```python
from build123d import *

# Parameters (mm, degrees)
F0_W      = 298.5
F0_H      = 130
F1_DEPTH  = 14
F2_W      = 20
F2_H      = 10
F3_DEPTH  = 130
F4_W      = 11
F4_H      = 16
F5_DEPTH  = 130
F6_W      = 39.1095238095
F6_H      = 26.9544340008
F6_W_2    = 43.7704761905
F6_H_2    = 58.0455659992
F7_DEPTH  = 25
F8_R      = 2.5
F9_DEPTH  = 25
F10_R     = 2.5
F11_DEPTH = 318.501
F12_SIZE  = 3.49999
F14_W     = 276.5
F14_H     = 15
F13_DEPTH = 25


# Not quite as in the source:
# - a fillet or chamfer is up to 0.001 mm smaller than in the source, because OpenCascade refuses the exact size
# - a feature names something its author has since deleted; it is built from what else it names


with BuildPart() as f1:
    # F0 (on Front) → F1 (new body)
    with BuildSketch(Plane.XZ):
        with Locations((149.25, 65)):
            Rectangle(F0_W, F0_H)
    extrude(amount=F1_DEPTH)

    # F2 (on face) → F3 (join, through all)
    with BuildSketch(Plane.XY.offset(130)):
        with Locations((308.5, -9)):
            Rectangle(F2_W, F2_H)
        with Locations((-10, -9)):
            Rectangle(F2_W, F2_H)
    extrude(amount=-F3_DEPTH)

    # F4 (on face) → F5 (join, through all)
    with BuildSketch(Plane.XY.offset(130)):
        with Locations((5.5, 8)):
            Rectangle(F4_W, F4_H)
        with Locations((293, 8)):
            Rectangle(F4_W, F4_H)
    extrude(amount=-F5_DEPTH)

    # F6 (on face) → F7 (cut)
    with BuildSketch(Plane.XZ.offset(14)):
        Polygon((51.37, 120), (51.37, 93.0455659992), (36.37, 93.0455659992), (36.3699999999, 56.9544340008), (90.4795238095, 56.9544340008), (90.4795238095, 120), align=None)
        with Locations((70.9247619048, 28.4772170004)):
            Rectangle(F6_W, F6_H)
        with Locations((127.3647619048, 44.0227829996)):
            Rectangle(F6_W_2, F6_H_2)
        with Locations((171.1352380952, 44.0227829996)):
            Rectangle(F6_W_2, F6_H_2)
        with Locations((127.3647619048, 106.5227829996)):
            Rectangle(F6_W_2, F6_H)
        with Locations((171.1352380952, 106.5227829996)):
            Rectangle(F6_W_2, F6_H)
        Polygon((247.1300000001, 120), (208.0204761905, 120), (208.0204761905, 56.9544340008), (262.13, 56.9544340008), (262.13, 93.0455659992), (247.13, 93.0455659992), align=None)
        with Locations((227.5752380952, 28.4772170004)):
            Rectangle(F6_W, F6_H)
    extrude(amount=-F7_DEPTH, mode=Mode.SUBTRACT)

    # F8 (on face) → F9 (cut)
    with BuildSketch(Plane(origin=(0, -4, 0), x_dir=(-1, 0, 0), z_dir=(0, 1, 0))):
        with Locations((-298.5, 115)):
            Circle(F8_R)
        with Locations((-298.5, 15)):
            Circle(F8_R)
        with Locations((0, 115)):
            Circle(F8_R)
        with Locations((0, 15)):
            Circle(F8_R)
    extrude(amount=-F9_DEPTH, mode=Mode.SUBTRACT)

    # F10 (on face) → F11 (cut, through all)
    with BuildSketch(Plane.YZ.offset(298.5)):
        with Locations((6, 115)):
            Circle(F10_R)
        with Locations((6, 15)):
            Circle(F10_R)
        with Locations((6, 65)):
            Circle(F10_R)
    extrude(amount=-F11_DEPTH, mode=Mode.SUBTRACT)

    # F12 (size 3.5 in the source; OpenCascade refuses exactly that, so slightly less here)
    f12_edges = [f1.edges().sort_by_distance(p)[0] for p in [
        (301, -14, 115),
        (301, -14, 15),
        (2.5, -14, 115),
        (2.5, -14, 15),
        (287.5, 3.5, 115),
        (287.5, 3.5, 65),
        (287.5, 3.5, 15),
        (11, 3.5, 115),
        (11, 3.5, 65),
        (11, 3.5, 15),
    ]]
    chamfer(f12_edges, length=F12_SIZE)

    # F14 (on face) → F13 (join)
    with BuildSketch(Plane(origin=(0, 0, 0), x_dir=(-1, 0, 0), z_dir=(0, 1, 0))):
        with Locations((-149.25, 7.5)):
            Rectangle(F14_W, F14_H)
    extrude(amount=F13_DEPTH)


solid = f1.part
```
Verification items for the finished model (mm, model axes). A direction names the side the tool comes from. Coordinates: 2 decimals unless noted, no trailing zeros. Write each loop counter-clockwise with the first axis right and the second up, starting at its lowest first coordinate (ties: lowest second). Pieces come first, ordered by that corner, then holes. Notation, with made-up numbers: M -27,12 L 25,12 A23 cw 25,26 Z; hole C -33,47.25 d6. An arc over 180 degrees is marked long. One line per item, written item: value.
Item 1: Section check B-B, the plane z = 105.5. Record the boundary of the cut face in (x, y), plus the area to 3 significant figures.
Check sheet entries:
outline: M -20,-14 L 51.37,-14 L 51.37,0 L 11,0 L 11,16 L 0,16 L 0,-4 L -20,-4 Z; M 90.48,-14 L 105.48,-14 L 105.48,0 L 90.48,0 Z; M 193.02,-14 L 208.02,-14 L 208.02,0 L 193.02,0 Z; M 247.13,-14 L 318.5,-14 L 318.5,-4 L 298.5,-4 L 298.5,16 L 287.5,16 L 287.5,0 L 247.13,0 Z
area: 2,610 mm^2
Item 2: Scan lines: line 1 along Z through (x, y) = (1.5, 6); line 2 along X through (y, z) = (-10, 88.5); line 3 along Z through (x, y) = (0, -8). Record each from-to range of solid material in increasing order.
Check sheet entries:
line 1: z = 0 to 12.5, 17.5 to 62.5, 67.5 to 112.5, 117.5 to 130
line 2: x = -20 to 36.37, 90.48 to 208.02, 262.13 to 318.5
line 3: z = 0 to 12.5, 17.5 to 112.5, 117.5 to 130
Item 3: Access from +Z, -Z, +X, -X, +Y, -Y to the whole of each face (thin tool, end or side, straight path). Record for faces 4 (the flat face through (184, -5, 130)), 5 (the flat face through (90.48, -7, 88)), 6 (the conical face through (290.83, 7.44, 17.25)).
Check sheet entries:
face 4: +Z, +X, -X, +Y, -Y
face 5: +Y, -Y
face 6: none
Item 4: Section check A-A, the plane x = 239. Record the boundary of the cut face in (y, z).
Check sheet entries:
outline: M -14,0 L 25,0 L 25,15 L -14,15 Z; M -14,41.95 L 0,41.95 L 0,56.95 L -14,56.95 Z; M -14,120 L 0,120 L 0,130 L -14,130 Z
Item 5: Mould release check, pull along X, two halves, no side actions. Record for faces 1 (the flat face through (11, 20, 7)), 2 (the flat face through (5, 16, 66)), 3 (the flat face through (247.13, -7, 28)): pulls with the +X half, pulls with the -X half, needs draft (parallel to the pull), parting line crosses it, or undercut.
Check sheet entries:
face 1: pulls with the -X half
face 2: needs draft
face 3: undercut
Item 6: Section check C-C, the plane x = 168.5. Record the boundary of the cut face in (y, z).
Check sheet entries:
outline: M -14,0 L 25,0 L 25,15 L -14,15 Z; M -14,73.05 L 0,73.05 L 0,93.05 L -14,93.05 Z; M -14,120 L 0,120 L 0,130 L -14,130 Z
Item 7: Gauge pin test, flat ends, axial feed: pin 1 Ø16 at (y, z) = (9, 96) entering from +X; pin 2 Ø3 at (y, z) = (6, 115) entering from +X; pin 3 Ø4 at (x, y) = (241, 10.5) entering from +Z; pin 4 Ø3 at (x, z) = (296.5, 115) entering from -Y. Record the tip position at first contact, or that the pin passes through.
Check sheet entries:
pin 1: stops at x = 298.5
pin 2: passes through
pin 3: stops at z = 15
pin 4: stops at y = -11.5
